Autodesk Inventor part; units mm, degrees
ref_plane "YZ Plane" through (0, 0, 0) normal (1, 0, 0) x (0, 1, 0)
ref_plane "XZ Plane" through (0, 0, 0) normal (0, 1, 0) x (-1, 0, 0)
ref_plane "XY Plane" through (0, 0, 0) normal (0, 0, 1) x (1, 0, 0)
sketch "Sketch1" plane through (0, 0, 0) normal (0, 0, 1) x (1, 0, 0)
  line L0 (0, 0) -> (25.4, 0)
  line L1 (25.4, 0) -> (25.4, 25.4)
  line L2 (25.4, 25.4) -> (0, 25.4)
  line L3 (0, 25.4) -> (0, 0)
  line L4 (1.5875, 1.5875) -> (23.8125, 1.5875)
  line L5 (23.8125, 1.5875) -> (23.8125, 23.8125)
  line L6 (23.8125, 23.8125) -> (1.5875, 23.8125)
  line L7 (1.5875, 23.8125) -> (1.5875, 1.5875)
  dimension "d0" = 25.4
  dimension "d1" = 25.4
  dimension "d2" = 1.5875
extrude "Extrusion1" add sketch "Sketch1" along normal blind 400.05
sketch "Sketch3" plane through (0, 25.4, 0) normal (0, 1, 0) x (1, 0, 0)
  line L0 (25.4, 0) -> (0, 0)
  line L1 (0, 0) -> (0, -400.05)
  line L2 (25.4, -400.05) -> (0, -400.05)
  line L3 (25.4, 0) -> (25.4, -400.05)
  point P0 (0, 0)
  point P1 (12.7, -200.025)
  dimension "d15" = 200.025
  dimension "d16" = 400.05
  dimension "d17" = 12.7
hole "Hole2" at (12.7, 25.4, 200.025) direction (0, -1, 0) diameter 6.35 end through all
sketch "Sketch5" plane through (0, 25.4, 0) normal (0, 1, 0) x (1, 0, 0)
  line L0 (0, 0) -> (0, -400.05)
  line L1 (25.4, -400.05) -> (0, -400.05)
  point P0 (12.7, -387.35)
  dimension "d25" = 12.7
  dimension "d26" = 12.7
hole "Hole3" at (12.7, 25.4, 387.35) direction (0, -1, 0) diameter 4.8514 end through all
pattern_linear "Rectangular Pattern1" count 3 spacing 19.05 along (0, 0, -1) of "Hole3"
sketch "Sketch6" plane through (0, 25.4, 0) normal (0, 1, 0) x (1, 0, 0)
  line L0 (25.4, 0) -> (0, 0)
  line L1 (25.4, 0) -> (25.4, -400.05)
  point P0 (12.7, -12.7)
  dimension "d37" = 12.7
  dimension "d38" = 12.7
hole "Hole4" at (12.7, 25.4, 12.7) direction (0, -1, 0) diameter 4.8514 end through all
pattern_linear "Rectangular Pattern2" count 3 spacing 19.05 along (0, 0, 1) of "Hole4"
properties part number "CLB_043_FourPartScissorBarMiddle" material "Aluminum 6061"
Input: part model. Units: mm. Frame: model coordinates. A direction names the side the tool comes from. Give positions to 0.01 mm unless a question says otherwise; leave off trailing zeros. Write each loop counter-clockwise with the first axis right and the second up, starting at its lowest first coordinate (ties: lowest second). Pieces come first, ordered by that corner, then holes. Notation, with made-up numbers: M -13.5,-40 L 25.5,-40 A24 cw 25.5,-7 Z; hole C -35,63.25 d9. An arc over 180 degrees is marked long. Write item = value, one per line. Start each with the question number.
1) Cut plane A-A on x = 20.5. Return the cut outline in (y, z).
2) Material intervals for line 1 along X through (y, z) = (0.65, 31.75); line 2 along X through (y, z) = (18.5, 247), sorted ascending. Write a range as [from, to].
3) Cut plane C-C on z = 246.5. Return the cut outline in (x, y).
4) First-contact query: pin 1 Ø12 at (y, z) = (8, 343.5) entering from -X; pin 2 Ø6 at (x, y) = (5, 5.5) entering from -Z. Flat tips, straight axial feed; report the tip coordinate or a pass-through.
5) Draft query along X for faces 3 (the flat face through (0, 13, 197)), 4 (the flat face through (23.812, 13, 197)), 5 (the flat face through (25.4, 13, 197)). Return one class per face: +X half, -X half, draft (parallel to the pull), parting line (faces both ways), or undercut.
6) Reachability of faces 1 (the flat face through (15, 0, 197)), 2 (the flat face through (1.588, 13, 197)) from +Z, -Z, +X, -X, +Y, -Y: full face, straight path, thin tool, end or side. Return the list, or none.
Solved:
q1.outline = M 0,0 L 1.59,0 L 1.59,400.05 L 0,400.05 Z; M 23.81,0 L 25.4,0 L 25.4,400.05 L 23.81,400.05 Z
q2.line_1 = [0, 10.27], [15.13, 25.4]
q2.line_2 = [0, 1.59], [23.81, 25.4]
q3.outline = M 0,0 L 25.4,0 L 25.4,25.4 L 0,25.4 Z; hole M 1.59,1.59 L 23.81,1.59 L 23.81,23.81 L 1.59,23.81 Z
q4.pin_1 = 0
q4.pin_2 = through
q5.face_3 = -X half
q5.face_4 = undercut
q5.face_5 = +X half
q6.face_1 = +Z, -Z, +X, -X, -Y
q6.face_2 = +Z, -Z
